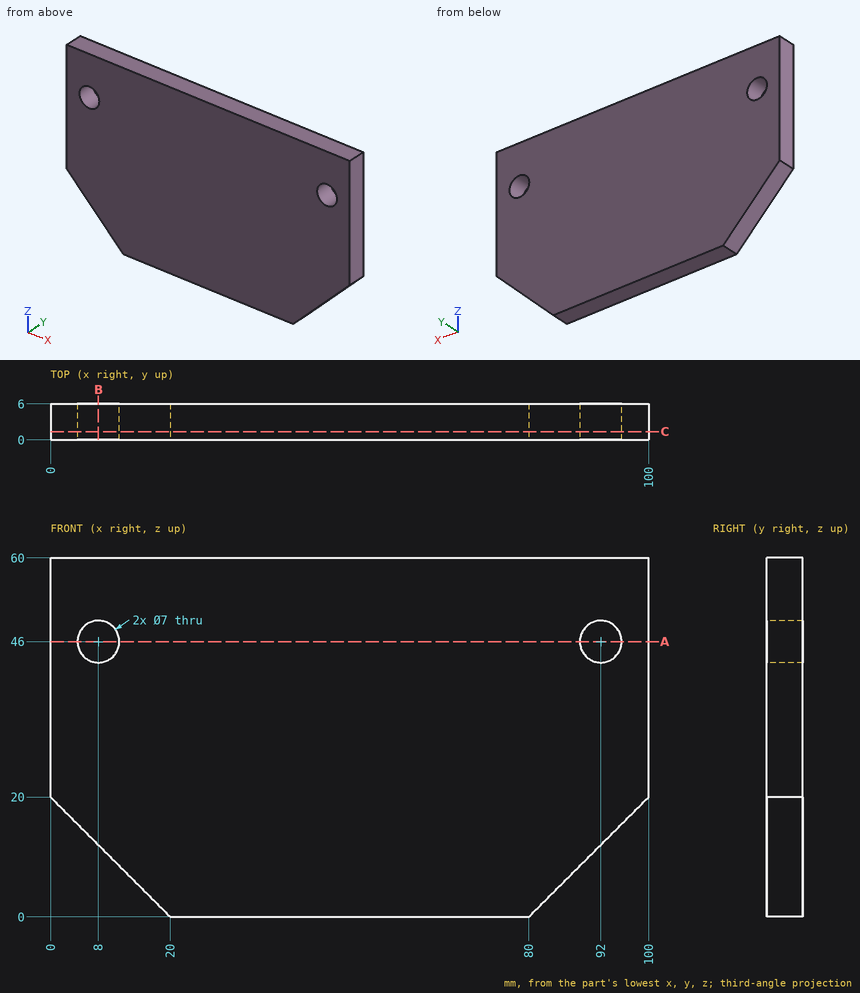
Study the drawing (mm; zero at the part's minimum x, y, z) and answer. Round coordinates to 2 decimals unless told otherwise and drop trailing zeros. Write each loop counter-clockwise with the first axis right and the second up, starting at its lowest first coordinate (ties: lowest second). Pieces come first, ordered by that corner, then holes. Notation, with made-up numbers: (71, 84) -> (98, 84) arc R27 ccw to (98, 116) -> close; hole circle Ø2 at (-7.75, 74). An arc over 180 degrees is marked (long way). Write each question's results on one line, items separated by ' | '.
Item 1: A cutting plane is placed at B-B, the plane x = 8. Determine the outline of the cut face in (y, z), plus the area to 3 significant figures.
Result set:
outline: (0, 12) -> (6, 12) -> (6, 42.5) -> (0, 42.5) -> close; (0, 49.5) -> (6, 49.5) -> (6, 60) -> (0, 60) -> close | area: 246 mm^2
Item 2: A cutting plane is placed at A-A, the plane z = 46. Determine the outline of the cut face in (x, y), plus the area to 3 significant figures.
Result set:
outline: (0, 0) -> (4.5, 0) -> (4.5, 6) -> (0, 6) -> close; (11.5, 0) -> (88.5, 0) -> (88.5, 6) -> (11.5, 6) -> close; (95.5, 0) -> (100, 0) -> (100, 6) -> (95.5, 6) -> close | area: 516 mm^2
Item 3: Find the intervals of material crossed by line 1 along X through (y, z) = (2, 49); line 2 along Z through (x, y) = (8, 3.2); line 3 along X through (y, z) = (2.85, 8), in increasing order. Write a range as [from, to].
Result set:
line 1: [0, 6.2], [9.8, 90.2], [93.8, 100] | line 2: [12, 42.5], [49.5, 60] | line 3: [12, 88]
Item 4: A cutting plane is placed at C-C, the plane y = 1.4. Determine the outline of the cut face in (x, z).
Result set:
outline: (0, 20) -> (20, 0) -> (80, 0) -> (100, 20) -> (100, 60) -> (0, 60) -> close; hole circle Ø7 at (8, 46); hole circle Ø7 at (92, 46)
